Part model, mm, in its own coordinate system. Face numbers are marked on the shaded views. Give positions to 0.01 mm unless a question says otherwise; leave off trailing zeros. Order: outer loops, then holes, each group sorted by start corner. A loop starts at its lowest first (then second) coordinate and runs counter-clockwise, first axis right, second up.
1. Mould opens along Z. For the marked faces 1 and 2 say: +Z half, -Z half, draft (parallel to the pull), parting line (faces both ways), or undercut.
2. Drop a flat-ended pin along its axis: pin 1 Ø1 at (x, y) = (-4.5, -3) entering from -Z. Give the stop position or say it passes through.
3. Slice it at B-B on x = -4. Give the number of separate pieces and of enclosed holes in the cut face, and give its area (3 significant figures).
4. Slice it at A-A on z = 0. List the corners of the cut face in (x, y).
5. Probe line 1 (Z direction, x = 0, y = -3.2); line 2 (Z direction, x = -1.5, y = -1.9); line 3 (Z direction, x = 7.5, y = -2.3). List the from-to ranges inside material, lowest first.
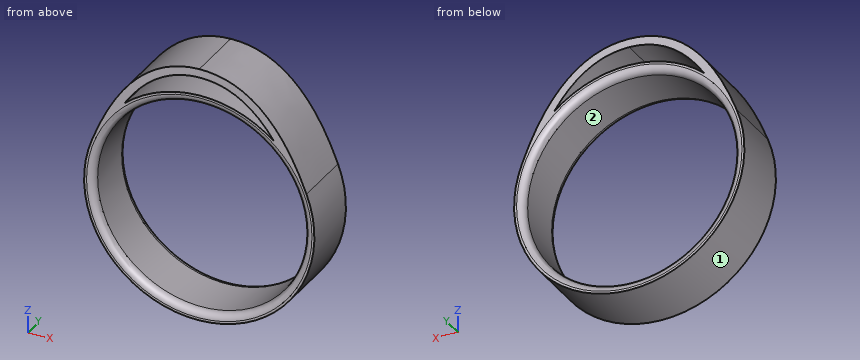
from build123d import *

# Parameters (mm, degrees)
F0_R     = 9.4
F0_R_2   = 8.6
F1_DEPTH = 5
F3_DEPTH = 5
F4_R     = 0.6


# Not quite as in the source:
# - the dataset's text gives a spline's control points without its knots; the knots are read off the source's solid


with BuildPart() as f1:
    # F0 (on Front) → F1 (new body)
    with BuildSketch(Plane.XZ):
        Circle(F0_R)
        Circle(F0_R_2, mode=Mode.SUBTRACT)
    extrude(amount=F1_DEPTH)

    # F2 (on Front) → F3 (join)
    with BuildSketch(Plane.XZ):
        with BuildLine():
            add(Edge.make_bspline(
                [(-8.8490276873, 3.1709161121), (-7.3496829409, 7.2272375548), (-4.746891386, 11.5964177027), (3.78631e-05, 11.5964002776), (5.67948e-05, 11.5964002775)],
                knots=[0, 0, 0, 0, 0.5, 0.5000019941, 0.5000019941, 0.5000019941, 0.5000019941], degree=3))
            Line((-8.8490276873, 3.1709161121), (-8.1924457198, 2.9282226429))
            add(Edge.make_bspline(
                [(-8.1924457198, 2.9282226429), (-7.8262756691, 3.9188576733), (-6.9626502108, 5.9278467604), (-5.4967702335, 8.1305819439), (-4.0755610615, 9.4931807293), (-2.8820227839, 10.2720641504), (-1.7694285607, 10.6893985819), (-0.7912754674, 10.8653850416), (-0.2703531008, 10.896417707), (0, 10.8964002777)],
                knots=[0, 0, 0, 0, 0.125, 0.25, 0.3125, 0.375, 0.4375, 0.46875, 0.5, 0.5, 0.5, 0.5], degree=3))
            add(Edge.make_bspline(
                [(8.1924457198, 2.9282226429), (7.8262756691, 3.9188576733), (6.9626502108, 5.9278467604), (5.4967702335, 8.1305819439), (4.0755610615, 9.4931807293), (2.8820227839, 10.2720641504), (1.7694285607, 10.6893985819), (0.7912754674, 10.8653850416), (0.2703531008, 10.896417707), (0, 10.8964002777)],
                knots=[0, 0, 0, 0, 0.125, 0.25, 0.3125, 0.375, 0.4375, 0.46875, 0.5, 0.5, 0.5, 0.5], degree=3))
            Line((8.1924457198, 2.9282226429), (8.8490276873, 3.1709161121))
            add(Edge.make_bspline(
                [(8.8490276873, 3.1709161121), (7.3496889206, 7.2272213774), (4.7469225273, 11.5963654275), (5.67948e-05, 11.5964002775)],
                knots=[0, 0, 0, 0, 0.4999980059, 0.4999980059, 0.4999980059, 0.4999980059], degree=3))
        make_face()
    extrude(amount=F3_DEPTH)

    # F4
    f4_edges = [f1.edges().sort_by_distance(p)[0] for p in [
        (-8.6, -5, 0),
        (-8.6, 0, 0),
    ]]
    fillet(f4_edges, radius=F4_R)


solid = f1.part
Data:
1. face 1: parting line
1. face 2: undercut
2. pin 1: stops at z = -8.51
3. separate pieces: 3
3. enclosed holes: 0
3. area: 12.9 mm2
4. outline: (-9.4, -5) - (-9.2, -5) arc R0.6 ccw to (-8.6, -4.4) - (-8.6, -0.6) arc R0.6 ccw to (-9.2, 0) - (-9.4, 0) - close; (8.6, -4.4) arc R0.6 ccw to (9.2, -5) - (9.4, -5) - (9.4, 0) - (9.2, 0) arc R0.6 ccw to (8.6, -0.6) - close
5. line 1: z = -9.4 to -8.6, 8.6 to 9.4, 10.9 to 11.6
5. line 2: z = -9.28 to -8.47, 8.47 to 9.28, 10.72 to 11.44
5. line 3: z = -5.67 to -4.21, 4.21 to 6.2
